Source: CAD feature listing. Evaluate the final solid. Frame: model axes, mm. Face numbers are marked on the shaded views. A direction names the side the tool comes from. Round coordinates to 2 decimals unless told otherwise and drop trailing zeros. Write each loop counter-clockwise with the first axis right and the second up, starting at its lowest first coordinate (ties: lowest second). Pieces come first, ordered by that corner, then holes. Notation, with made-up numbers: M -39,76.5 L -22,76.5 A35 ccw -22,113.5 Z; hole C -28.75,18.5 d4. An arc over 180 degrees is marked long. Put each result on its own line as item: value. Start each with the question number.
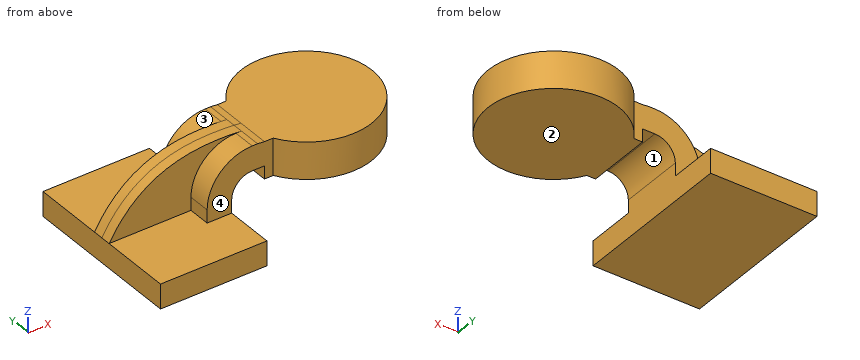
```python
from build123d import *

# Parameters (mm, degrees)
F1_DEPTH = 63.5
F2_DEPTH = 7.9375
F3_DEPTH = 25.4


with BuildPart() as f1:
    # F0 (on Front) → F1 (new body, symmetric)
    with BuildSketch(Plane.XZ):
        Polygon((22.225, 9.525), (-41.275, 9.525), (-41.275, -9.525), (41.275, -9.525), (41.275, 9.525), align=None)
    extrude(amount=F1_DEPTH, both=True)

    # F0 (on Front) → F2 (join, symmetric)
    with BuildSketch(Plane.XZ):
        with BuildLine():
            add(Edge.make_bspline(
                [(-41.275, 9.525), (-17.372467, 50.623456), (19.370141, 58.072404), (61.345564, 54.485139)],
                knots=[0, 0, 0, 0, 112.026415, 112.026415, 112.026415, 112.026415], degree=3))
            Line((-41.275, 9.525), (22.225, 9.525))
            Line((22.225, 9.525), (22.225, 19.560138))
            ThreePointArc((22.225, 19.560138), (32.454295, 44.255843), (57.15, 54.485139))
            Line((57.15, 54.485139), (61.345564, 54.485139))
        make_face()
    extrude(amount=F2_DEPTH, both=True)

    # F0 (on Front) → F3 (join, symmetric)
    with BuildSketch(Plane.XZ):
        with BuildLine():
            Line((22.225, 19.560138), (22.225, 9.525))
            Line((22.225, 9.525), (41.275, 9.525))
            Line((41.275, 9.525), (41.275, 19.560138))
            ThreePointArc((41.275, 19.560138), (45.92468, 30.785458), (57.15, 35.435138))
            Line((57.15, 35.435138), (66.675, 35.435138))
            Line((66.675, 35.435138), (66.675, 53.975))
            add(Edge.make_bspline(
                [(61.345564, 54.485139), (63.112955, 54.334095), (64.889623, 54.163487), (66.675, 53.975)],
                knots=[112.026415, 112.026415, 112.026415, 112.026415, 116.74333, 116.74333, 116.74333, 116.74333], degree=3))
            Line((61.345564, 54.485139), (57.15, 54.485139))
            ThreePointArc((57.15, 54.485139), (32.454295, 44.255843), (22.225, 19.560138))
        make_face()
        Polygon((117.475, 53.975), (66.675, 53.975), (66.675, 35.435138), (66.675, 25.4), (117.475, 25.4), align=None)
    extrude(amount=F3_DEPTH, both=True)

    # F0 (on Front) → F4 (revolve)
    with BuildSketch(Plane.XZ):
        Polygon((117.475, 53.975), (66.675, 53.975), (66.675, 35.435138), (66.675, 25.4), (117.475, 25.4), align=None)
    revolve(axis=Axis((117.475, 0, 39.6875), (0, 0, -1)))


solid = f1.part
```
(1) Section query A-A (y = 42). Return loops of the section in (x, z) (3 decimals).
(2) Ray query, line 1 along X through (y, z) = (-27.5, -2) (3 decimals); line 2 along Z through (x, y) = (122, 24) (3 decimals); line 3 along Z through (x, y) = (33.5, -53) (3 decimals). Return the intervals inside material, ascending.
(3) Section query B-B (x = 107.5). Return loops of the section in (y, z) (3 decimals).
(4) Access query for the marked faces 1, 2, 3 and 4. Directions: +Z, -Z, +X, -X, +Y, -Y. A direction counts if a zero-diameter tool reaches every point of the face in a straight line with its end or side. Return the directions, or none.
(5) Contact query for flat-ended pins moving along their axis: P1, Ø4, axis at x = 132.5, y = 38, coming from the +Z side (3 decimals); P2, Ø16.5, axis at x = 20, y = 35.5, coming from the +Z side (3 decimals); P3, Ø13.5, axis at x = 54, z = 34.5, coming from the +Y side. Output: stop coordinate, or through.
Entries:
1. outline: M -41.275,-9.525 L 41.275,-9.525 L 41.275,9.525 L -41.275,9.525 Z; M 88.898,25.4 L 146.052,25.4 L 146.052,53.975 L 88.898,53.975 Z
2. line 1: -41.275 to 41.275
2. line 2: 25.4 to 53.975
2. line 3: -9.525 to 9.525
3. outline: M -49.811,25.4 L 49.811,25.4 L 49.811,53.975 L -49.811,53.975 Z
4. face 1: -Z, +Y, -Y
4. face 2: -Z, +X, +Y, -Y
4. face 3: +Z, -X, +Y
4. face 4: +Z, -X, -Y
5. P1: z = 53.975
5. P2: z = 9.525
5. P3: y = 25.4
